```python
from build123d import *

# Parameters (mm, degrees)
SKETCH_2_W          = 23.4
SKETCH_2_H          = 7.4
SKETCH_2_W_2        = 7.4
SKETCH_2_H_2        = 23.4
EXTRUDE_1_DEPTH     = 7.8
EXTRUDE_START       = -1
SKETCH_3_W          = 14.4
SKETCH_3_H          = 12.4
EXTRUDE_2_DEPTH     = 5
SKETCH_2_6_R        = 2.5
SKETCH_2_6_R_2      = 3.5
CUT_EXTRUDE_3_DEPTH = 19.292621463
SKETCH_2_3_R        = 3.15
CUT_EXTRUDE_1_DEPTH = 1
CUT_EXTRUDE_START   = 6.8
SKETCH_2_5_R        = 3.15
CUT_EXTRUDE_2_DEPTH = 1
SKETCH_4_R          = 0.8
CUT_EXTRUDE_4_DEPTH = 21.322893495
SKETCH_2_7_R        = 3.5
SKETCH_2_7_R_2      = 3.15
CUT_EXTRUDE_5_DEPTH = 19.292621463


with BuildPart() as part:
    # 草图2 → 凸台-拉伸1 (new body)
    with BuildSketch(Plane.XY):
        Rectangle(SKETCH_2_W, SKETCH_2_H)
        Rectangle(SKETCH_2_W_2, SKETCH_2_H_2)
    extrude(amount=EXTRUDE_1_DEPTH)

    # 草图3 → 凸台-拉伸2 (add)
    with BuildSketch(Plane(origin=(0, 0, 0), x_dir=(-1, 0, 0), z_dir=(0, 0, -1)).offset(EXTRUDE_START)):
        Rectangle(SKETCH_3_W, SKETCH_3_H)
    extrude(amount=EXTRUDE_2_DEPTH)

    # 草图2<6> → 切除-拉伸3 (cut, through all)
    with BuildSketch(Plane.XY):
        with BuildLine():
            Line((-3.7, 11.7), (-3.7, 8))
            ThreePointArc((-3.7, 8), (-2.61629509, 10.61629509), (0, 11.7))
            Line((0, 11.7), (-3.7, 11.7))
        make_face()
        with BuildLine():
            ThreePointArc((0, 11.7), (2.61629509, 10.61629509), (3.7, 8))
            Line((3.7, 8), (3.7, 11.7))
            Line((3.7, 11.7), (0, 11.7))
        make_face()
        with BuildLine():
            Line((11.7, 3.7), (8.000000006, 3.7))
            ThreePointArc((8.000000006, 3.7), (10.616295093, 2.616295088), (11.7, 0))
            Line((11.7, 0), (11.7, 3.7))
        make_face()
        with BuildLine():
            ThreePointArc((11.7, 0), (10.616295085, -2.616295096), (7.999999984, -3.7))
            Line((7.999999984, -3.7), (11.7, -3.7))
            Line((11.7, -3.7), (11.7, 0))
        make_face()
        with BuildLine():
            Line((3.7, -11.7), (3.7, -8))
            ThreePointArc((3.7, -8), (2.61629509, -10.61629509), (0, -11.7))
            Line((0, -11.7), (3.7, -11.7))
        make_face()
        with BuildLine():
            ThreePointArc((0, -11.7), (-2.616295094, -10.616295087), (-3.7, -7.99999999))
            Line((-3.7, -7.99999999), (-3.7, -11.7))
            Line((-3.7, -11.7), (0, -11.7))
        make_face()
        with BuildLine():
            Line((-11.7, -1.1e-08), (-11.7, -3.7))
            Line((-11.7, -3.7), (-8.000000004, -3.7))
            ThreePointArc((-8.000000004, -3.7), (-10.616295088, -2.616295093), (-11.7, -1.1e-08))
        make_face()
        with BuildLine():
            Line((-11.7, 3.7), (-11.7, -1.1e-08))
            ThreePointArc((-11.7, -1.1e-08), (-10.616295094, 2.616295086), (-8, 3.7))
            Line((-8, 3.7), (-11.7, 3.7))
        make_face()
        with Locations(Location((0, 8, 0), (0, 0, 226.054480438))):
            Circle(SKETCH_2_6_R)
        with Locations(Location((-8, 0, 0), (0, 0, 288.662924885))):
            Circle(SKETCH_2_6_R)
        Circle(SKETCH_2_6_R_2)
        with Locations(Location((8, 0, 0), (0, 0, 108.662924885))):
            Circle(SKETCH_2_6_R)
        with Locations(Location((0, -8, 0), (0, 0, 133.945519562))):
            Circle(SKETCH_2_6_R)
    extrude(amount=CUT_EXTRUDE_3_DEPTH, mode=Mode.SUBTRACT)

    # 草图2<3> → 切除-拉伸1 (cut)
    with BuildSketch(Plane.XY):
        with Locations(Location((8, 0, 0), (0, 0, 255.287542039))):
            Circle(SKETCH_2_3_R)
        with Locations(Location((-8, 0, 0), (0, 0, 284.712457961))):
            Circle(SKETCH_2_3_R)
        with Locations(Location((0, 8, 0), (0, 0, 214.849904579))):
            Circle(SKETCH_2_3_R)
        with Locations(Location((0, -8, 0), (0, 0, 145.150095421))):
            Circle(SKETCH_2_3_R)
    extrude(amount=CUT_EXTRUDE_1_DEPTH, mode=Mode.SUBTRACT)

    # 草图2<5> → 切除-拉伸2 (cut)
    with BuildSketch(Plane.XY.offset(CUT_EXTRUDE_START)):
        with Locations(Location((8, 0, 0), (0, 0, 255.287542039))):
            Circle(SKETCH_2_5_R)
        with Locations(Location((-8, 0, 0), (0, 0, 284.712457961))):
            Circle(SKETCH_2_5_R)
        with Locations(Location((0, 8, 0), (0, 0, 214.849904579))):
            Circle(SKETCH_2_5_R)
        with Locations(Location((0, -8, 0), (0, 0, 145.150095421))):
            Circle(SKETCH_2_5_R)
    extrude(amount=CUT_EXTRUDE_2_DEPTH, mode=Mode.SUBTRACT)

    # 草图4 → 切除-拉伸4 (cut, through all)
    with BuildSketch(Plane(origin=(0, 0, -4), x_dir=(-1, 0, 0), z_dir=(0, 0, -1))):
        with Locations((5.45, 4.95)):
            Circle(SKETCH_4_R)
        with Locations((-5.45, 4.95)):
            Circle(SKETCH_4_R)
        with Locations((5.45, -4.95)):
            Circle(SKETCH_4_R)
        with Locations((-5.45, -4.95)):
            Circle(SKETCH_4_R)
    extrude(amount=-CUT_EXTRUDE_4_DEPTH, mode=Mode.SUBTRACT)

    # 草图2<7> → 切除-拉伸5 (cut, through all)
    with BuildSketch(Plane.XY):
        Circle(SKETCH_2_7_R)
        with Locations(Location((8, 0, 0), (0, 0, 104.712457961))):
            Circle(SKETCH_2_7_R_2)
        with Locations(Location((-8, 0, 0), (0, 0, 284.712457961))):
            Circle(SKETCH_2_7_R_2)
        with Locations(Location((0, 8, 0), (0, 0, 214.849904579))):
            Circle(SKETCH_2_7_R_2)
        with Locations(Location((0, -8, 0), (0, 0, 145.150095421))):
            Circle(SKETCH_2_7_R_2)
    extrude(amount=-CUT_EXTRUDE_5_DEPTH, mode=Mode.SUBTRACT)


solid = part.part
```
The model under review builds one solid part; all positions refer to its coordinate system, in mm. A direction names the side the tool comes from. Coordinates: 2 decimals unless noted, no trailing zeros. Order: outer loops, then holes, each group sorted by start corner. A loop starts at its lowest first (then second) coordinate and runs counter-clockwise, first axis right, second up. Notation, with made-up numbers: M 53.5,51.5 L 87.5,51.5 A18 ccw 87.5,75.5 Z; hole C 62,69 d4. An arc over 180 degrees is marked long. One line per question, with ' | ' between items.
(1) Add section B-B, the plane y = -2. State how many separate pieces and enclosed holes the cut face has, then the cut area to 3 significant figures.
Geometry results:
separate pieces: 4 | enclosed holes: 0 | area: 95.8 mm²
(2) Add section A-A, the plane z = -2.75. Write out the cut boundary in (x, y), then the cut area to 3 significant figures.
Geometry results:
outline: M -7.2,-6.2 L -2.59,-6.2 A3.15 cw 2.59,-6.2 L 7.2,-6.2 L 7.2,-3.05 A3.15 cw 7.2,3.05 L 7.2,6.2 L 2.59,6.2 A3.15 cw -2.59,6.2 L -7.2,6.2 L -7.2,3.05 A3.15 cw -7.2,-3.05 Z; hole C -5.45,-4.95 d1.6; hole C -5.45,4.95 d1.6; hole C 0,0 d7; hole C 5.45,-4.95 d1.6; hole C 5.45,4.95 d1.6 | area: 101 mm²
(3) Insertion check: pin 1 (2 mm diameter, centred on y = -2, z = 0, fed in from -X); pin 2 (5 mm diameter, centred on x = 0, y = 7.5, fed in from -Z); pin 3 (0.9 mm diameter, centred on y = -4.5, z = -2, fed in from -X). Each pin has a flat end and moves straight along its axis. Give the tip position at first contact, or say it passes through.
Geometry results:
pin 1: stops at x = -11.56 | pin 2: stops at z = 1 | pin 3: stops at x = -7.2
(4) Machinability: for faces 3 (the face through (5, 6, 1)), 4 (the face through (-5, -4, 1)), 5 (the face through (3, 8, 6.8)), 6 (the face through (3, 8, 1)), which of the approach directions +Z, -Z, +X, -X, +Y, -Y give a long, thin tool a straight path to every point of the face, cutting with its end or side? Answer none if there is none.
Geometry results:
face 3: +Z, +X, +Y | face 4: +Z, -X, -Y | face 5: +Z | face 6: -Z
(5) The part is to be moulded in two halves that separate along Y. For faces 1 (the face through (-11.148, -0.121, 7.293)), 2 (the face through (-3.7, -6, 4)), say which applies: +Y half, -Y half, draft (parallel to the pull), parting line (faces both ways), or undercut.
Geometry results:
face 1: undercut | face 2: draft
(6) Add section D-D, the plane x = 4. Write out the cut boundary in (y, z).
Geometry results:
outline: M -6.2,-4 L 6.2,-4 L 6.2,1 L 3.7,1 L 3.7,7.8 L -3.7,7.8 L -3.7,1 L -6.2,1 Z
(7) For probe 1 along Y at (x, z) = (-8, 5.5); probe 2 along Y at (x, z) = (1, 1.75); probe 3 along X at (y, z) = (8, 7.45), list the stretches that pass through material, from the lowest coordinate up. Write a range as from..to.
Geometry results:
probe 1: y = -3.7..-2.5, 2.5..3.7 | probe 2: y = -11.56..-10.29, -5.71..-3.35, 3.35..5.71, 10.29..11.56 | probe 3: x = -3.7..-3.15, 3.15..3.7
(8) Add section C-C, the plane y = -10. Write out the cut boundary in (x, z).
Geometry results:
outline: M -3.11,0 L -2.43,0 L -2.43,1 L -1.5,1 L -1.5,6.8 L -2.43,6.8 L -2.43,7.8 L -3.11,7.8 Z; M 1.5,1 L 2.43,1 L 2.43,0 L 3.11,0 L 3.11,7.8 L 2.43,7.8 L 2.43,6.8 L 1.5,6.8 Z
